Design review of the part built by this model. Coordinates are the model's own, in mm. A direction names the side the tool comes from. Coordinates: 2 decimals unless noted, no trailing zeros. Loops run counter-clockwise (first coordinate to the right, second up) from the corner with the lowest first, then second, coordinate; pieces in that order, holes last. Notation, with made-up numbers: (27.25, 4) - (46.25, 4) arc R20 cw to (46.25, 35) - close; hole circle Ø10 at (28.5, 82.5). An arc over 180 degrees is marked (long way). Return JSON: item names as keys, results as strings. Group by question number.
from build123d import *

# Parameters (mm, degrees)
EXTRUDE_1_DEPTH      = 39
SKETCH_2_R           = 5.5
CUT_EXTRUDE_1_DEPTH  = 5
SKETCH_3_R           = 2.75
CUT_EXTRUDE_2_DEPTH  = 25.5
SKETCH_4_R           = 2.1
CUT_EXTRUDE_3_DEPTH  = 30
HOLEWZD1_D           = 8.2
HOLEWZD1_DEPTH       = 16
HOLEWZD1_CSINK_D     = 8.5
HOLEWZD1_CSINK_ANGLE = 82
CHAMFER1_SIZE        = 0.5


with BuildPart() as part:
    # Эскиз1 → Бобышка-Вытянуть1 (new body, symmetric)
    with BuildSketch(Plane.XY):
        with BuildLine():
            Line((74, -50), (74, -36))
            Line((74, -36), (55, -36))
            Line((55, -36), (55, 29))
            Line((55, 29), (40.730823709, 29))
            ThreePointArc((40.730823709, 29), (0, 50), (-40.730823709, 29))
            Line((-40.730823709, 29), (-55, 29))
            Line((-55, 29), (-55, 1.5))
            Line((-55, 1.5), (-39.971865105, 1.5))
            ThreePointArc((-39.971865105, 1.5), (40, 0), (-39.971865105, -1.5))
            Line((-39.971865105, -1.5), (-55, -1.5))
            Line((-55, -1.5), (-55, -36))
            Line((-55, -36), (-74, -36))
            Line((-74, -36), (-74, -50))
            Line((-74, -50), (74, -50))
        make_face()
    extrude(amount=EXTRUDE_1_DEPTH, both=True)

    # Эскиз2 → Вырез-Вытянуть1 (cut)
    with BuildSketch(Plane(origin=(0, 29, 0), x_dir=(1, 0, 0), z_dir=(0, 1, 0))):
        with Locations((-47.865411854, 30)):
            Circle(SKETCH_2_R)
        with Locations((-47.865411854, 0)):
            Circle(SKETCH_2_R)
        with Locations((-47.865411854, -30)):
            Circle(SKETCH_2_R)
    extrude(amount=-CUT_EXTRUDE_1_DEPTH, mode=Mode.SUBTRACT)

    # Эскиз3 → Вырез-Вытянуть2 (cut)
    with BuildSketch(Plane(origin=(0, 24, 0), x_dir=(1, 0, 0), z_dir=(0, 1, 0))):
        with Locations((-47.865411854, 30)):
            Circle(SKETCH_3_R)
        with Locations((-47.865411854, 0)):
            Circle(SKETCH_3_R)
        with Locations((-47.865411854, -30)):
            Circle(SKETCH_3_R)
    extrude(amount=-CUT_EXTRUDE_2_DEPTH, mode=Mode.SUBTRACT)

    # Эскиз4 → Вырез-Вытянуть3 (cut)
    with BuildSketch(Plane(origin=(0, -1.5, 0), x_dir=(1, 0, 0), z_dir=(0, 1, 0))):
        with Locations((-47.865411854, 30)):
            Circle(SKETCH_4_R)
        with Locations((-47.865411854, 0)):
            Circle(SKETCH_4_R)
        with Locations((-47.865411854, -30)):
            Circle(SKETCH_4_R)
    extrude(amount=-CUT_EXTRUDE_3_DEPTH, mode=Mode.SUBTRACT)

    # HoleWzd1
    with Locations(Plane(origin=(0, -36, 0), x_dir=(1, 0, 0), z_dir=(0, 1, 0))):
        with Locations((-64.5, 29), (-64.5, 0), (-64.5, -29), (64.5, -29), (64.5, 0), (64.5, 29)):
            CounterSinkHole(HOLEWZD1_D / 2, HOLEWZD1_CSINK_D / 2, depth=HOLEWZD1_DEPTH, counter_sink_angle=HOLEWZD1_CSINK_ANGLE)

    # Chamfer1
    chamfer1_edges = [part.edges().sort_by_distance(p)[0] for p in [
        (-47.865411854, 29, 39),
        (55, -3.5, -39),
        (64.5, -36, -39),
        (74, -43, -39),
        (0, -50, -39),
        (-55, 15.25, 39),
        (-74, -43, -39),
        (-64.5, -36, -39),
        (-55, -18.75, -39),
        (-47.485932553, -1.5, -39),
        (40, 0, -39),
        (-47.485932553, 1.5, -39),
        (-55, 15.25, -39),
        (-47.485932553, 1.5, 39),
        (-47.865411854, 29, -39),
        (0, 50, -39),
        (47.865411854, 29, -39),
        (40, 0, 39),
        (55, 29, 0),
        (55, -36, 0),
        (74, -36, 0),
        (74, -50, 0),
        (-74, -50, 0),
        (-74, -36, 0),
        (-55, -36, 0),
        (-55, -1.5, 0),
        (-55, 1.5, 0),
        (-55, 29, 0),
        (-47.485932553, -1.5, 39),
        (-55, -18.75, 39),
        (-64.5, -36, 39),
        (47.865411854, 29, 39),
        (-74, -43, 39),
        (0, -50, 39),
        (74, -43, 39),
        (64.5, -36, 39),
        (55, -3.5, 39),
        (0, 50, 39),
    ]]
    chamfer(chamfer1_edges, length=CHAMFER1_SIZE)


solid = part.part
Item 1: For faces 1 (the face through (48, 29, 1)), 2 (the face through (-58, -36, 1)), 3 (the face through (-45.242, 12.908, -0.826)), 4 (the face through (-44, 1.5, 1)), list the 3-axis set-ups (+Z, -Z, +X, -X, +Y, -Y) from which the entire face can be reached by the end or side of a thin tool; tool diameter is ignored.
Item 2: Add section A-A (x = -64.5). State the section outline as (y, z) points, then the cut area to 3 significant figures.
Item 3: Add section B-B (z = 10). State the section outline as (x, y) points.
Item 4: To check wall thickness, follow line 1 (Z direction, x = -64.5, y = -38.75); line 2 (X direction, y = -13, z = -29); line 3 (X direction, y = 10, z = -31.5). State the ranges of each line that lie inside material, in increasing order. Write a range as from..to.
Item 5: For P1, Ø9, axis at x = -47.87, z = 0, coming from the +Y side; P2, Ø1.5, axis at y = 16.5, z = -10, coming from the -X side; P3, Ø4, axis at x = -31, z = -3, coming from the +Y side, all flat-tipped, find the tip position at first contact; note any pin that passes through.
Item 6: Draft analysis for pull direction Y (two halves, no side actions). For faces 5 (the face through (-53.36, 26.54, 29.76)), 6 (the face through (0.665, 49.631, 38.865)), 7 (the face through (40.1, 1.74, 38.64)), state which applies: pulls with the +Y half, pulls with the -Y half, needs draft (parallel to the pull), parting line crosses it, or undercut.
Item 7: Add section C-C (x = 0). State the section outline as (y, z) points.
Item 8: Add section D-D (y = 10). Give the number of separate pieces and of enclosed holes in the cut face, then the cut area to 3 significant figures.
Answers below:
{
 "1": {"face 1": "+Z, -Z, +X, +Y", "face 2": "+Z, -Z, -X, +Y", "face 3": "+Y", "face 4": "+Z, -Z, -X"},
 "2": {"outline": "(-50, -38.5) - (-49.5, -39) - (-36.5, -39) - (-36, -38.5) - (-36, -33.25) - (-36.17, -33.1) - (-50, -33.1) - close; (-50, -24.9) - (-36.17, -24.9) - (-36, -24.75) - (-36, -4.25) - (-36.17, -4.1) - (-50, -4.1) - close; (-50, 4.1) - (-36.17, 4.1) - (-36, 4.25) - (-36, 24.75) - (-36.17, 24.9) - (-50, 24.9) - close; (-50, 33.1) - (-36.17, 33.1) - (-36, 33.25) - (-36, 38.5) - (-36.5, 39) - (-49.5, 39) - (-50, 38.5) - close", "area": "747 mm^2"},
 "3": {"outline": "(-74, -49.5) - (-73.5, -50) - (73.5, -50) - (74, -49.5) - (74, -36.5) - (73.5, -36) - (55.5, -36) - (55, -35.5) - (55, 28.5) - (54.5, 29) - (40.73, 29) arc R50 ccw to (-40.73, 29) - (-54.5, 29) - (-55, 28.5) - (-55, 2) - (-54.5, 1.5) - (-39.97, 1.5) arc R40 cw (long way) to (-39.97, -1.5) - (-54.5, -1.5) - (-55, -2) - (-55, -35.5) - (-55.5, -36) - (-73.5, -36) - (-74, -36.5) - close"},
 "4": {"line 1": "z = -39..-33.1, -24.9..-4.1, 4.1..24.9, 33.1..39", "line 2": "x = -55..-49.71, -46.02..-37.83, 37.83..55", "line 3": "x = -55..-50.17, -45.56..-38.73, 38.73..55"},
 "5": {"P1": "stops at y = 24", "P2": "stops at x = -55", "P3": "stops at y = 40.73"},
 "6": {"face 5": "needs draft", "face 6": "pulls with the +Y half", "face 7": "undercut"},
 "7": {"outline": "(-50, -38.5) - (-49.5, -39) - (-40.5, -39) - (-40, -38.5) - (-40, 38.5) - (-40.5, 39) - (-49.5, 39) - (-50, 38.5) - close; (40, -38.5) - (40.5, -39) - (49.5, -39) - (50, -38.5) - (50, 38.5) - (49.5, 39) - (40.5, 39) - (40, 38.5) - close"},
 "8": {"separate pieces": "2", "enclosed holes": "3", "area": "2,470 mm^2"}
}
